```python
from build123d import *
from build123d.topology import SkipClean

# Parameters (mm, degrees)
SKETCH1_W           = 152
SKETCH1_H           = 65.5
BOSS_EXTRUDE1_DEPTH = 44
SKETCH2_W           = 142
SKETCH2_H           = 25.5
CUT_EXTRUDE1_DEPTH  = 39
SKETCH4_W           = 60
SKETCH4_H           = 30
CUT_EXTRUDE2_DEPTH  = 30
BOSS_EXTRUDE3_REACH = 158.9
SKETCH5_W           = 10
SKETCH5_H           = 15
SKETCH9_W           = 152
SKETCH9_H           = 44
BOSS_EXTRUDE4_DEPTH = 10
CUT_EXTRUDE5_DEPTH  = 41.5
SKETCH11_W          = 142
SKETCH11_H          = 39
CUT_EXTRUDE6_DEPTH  = 5
SKETCH16_W          = 77
SKETCH16_H          = 25
CUT_EXTRUDE8_DEPTH  = 39
SKETCH17_R          = 10.5
CUT_EXTRUDE9_DEPTH  = 5
SKETCH18_R          = 7.5
CUT_EXTRUDE10_DEPTH = 5
SKETCH20_W          = 75.5
SKETCH20_H          = 44
BOSS_EXTRUDE6_DEPTH = 15
SKETCH21_W          = 10
SKETCH21_H          = 55.5
CUT_EXTRUDE12_DEPTH = 39
SKETCH22_W          = 20
SKETCH22_H          = 20
SKETCH22_W_2        = 7.5
SKETCH22_H_2        = 25
CUT_EXTRUDE13_DEPTH = 5
CUT_EXTRUDE14_DEPTH = 3.5
SKETCH24_W          = 5
SKETCH24_H          = 6.5
BOSS_EXTRUDE7_DEPTH = 5
SKETCH24_3_W        = 3
SKETCH24_3_H        = 12
BOSS_EXTRUDE8_DEPTH = 2.5
CUT_EXTRUDE7_DEPTH  = 6
BOSS_EXTRUDE5_DEPTH = 3
SKETCH19_R          = 2.35
SKETCH19_R_2        = 2.5
CUT_EXTRUDE11_DEPTH = 6
BOSS_EXTRUDE9_DEPTH = 40
CHAMFER1_SIZE       = 0.3


with BuildPart() as part:
    # Sketch1 → Boss-Extrude1 (new body)
    with BuildSketch(Plane(origin=(0, 0, 0), x_dir=(1, 0, 0), z_dir=(0, 1, 0))):
        Rectangle(SKETCH1_W, SKETCH1_H)
    extrude(amount=BOSS_EXTRUDE1_DEPTH)

    # Sketch2 → Cut-Extrude1 (cut)
    with BuildSketch(Plane(origin=(0, 44, 0), x_dir=(1, 0, 0), z_dir=(0, 1, 0))):
        with Locations((0, -20)):
            Rectangle(SKETCH2_W, SKETCH2_H)
    extrude(amount=-CUT_EXTRUDE1_DEPTH, mode=Mode.SUBTRACT)

    # Sketch4 → Cut-Extrude2 (cut)
    with BuildSketch(Plane(origin=(0, 44, 0), x_dir=(1, 0, 0), z_dir=(0, 1, 0))):
        with Locations((41, 7.75)):
            Rectangle(SKETCH4_W, SKETCH4_H)
    extrude(amount=-CUT_EXTRUDE2_DEPTH, mode=Mode.SUBTRACT)

    # Boss-Extrude3: up to this face of the body (flat: up to its plane)
    boss_extrude3_end = Plane(part.part.faces().sort_by_distance((71, 26.637767221, 6.817102138))[0])
    # Sketch5 → Boss-Extrude3 (add, up to the picked face)
    with BuildSketch(Plane(origin=(-71, 0, 0), x_dir=(0, 0, -1), z_dir=(1, 0, 0)), mode=Mode.PRIVATE) as boss_extrude3_sk1:
        with Locations((-12.25, 36.5)):
            Rectangle(SKETCH5_W, SKETCH5_H)
    boss_extrude3_tool1 = split(extrude(boss_extrude3_sk1.sketch, amount=BOSS_EXTRUDE3_REACH, mode=Mode.PRIVATE), bisect_by=boss_extrude3_end, keep=Keep.BOTH, mode=Mode.PRIVATE)
    add(boss_extrude3_tool1.solids().sort_by(Axis((-71, 36.5, 12.25), (1, 0, 0)))[0])

    # Sketch9 → Boss-Extrude4 (add)
    with BuildSketch(Plane.XY.offset(32.75)):
        with Locations((0, 22)):
            Rectangle(SKETCH9_W, SKETCH9_H)
    extrude(amount=BOSS_EXTRUDE4_DEPTH)

    # Sketch10 → Cut-Extrude5 (cut)
    with BuildSketch(Plane(origin=(0, 44, 0), x_dir=(1, 0, 0), z_dir=(0, 1, 0))):
        Polygon((-73.5, -32.75), (-73.5, -37.75), (73.5, -37.75), (73.5, -32.75), (71, -32.75), (-71, -32.75), align=None)
    extrude(amount=-CUT_EXTRUDE5_DEPTH, mode=Mode.SUBTRACT)

    # Sketch11 → Cut-Extrude6 (cut)
    with BuildSketch(Plane.XY.offset(42.75)):
        with Locations((0, 24.5)):
            Rectangle(SKETCH11_W, SKETCH11_H)
    extrude(amount=-CUT_EXTRUDE6_DEPTH, mode=Mode.SUBTRACT)

    # Sketch16 → Cut-Extrude8 (cut)
    with BuildSketch(Plane(origin=(0, 44, 0), x_dir=(1, 0, 0), z_dir=(0, 1, 0))):
        with Locations((-32.5, 10.25)):
            Rectangle(SKETCH16_W, SKETCH16_H)
    extrude(amount=-CUT_EXTRUDE8_DEPTH, mode=Mode.SUBTRACT)

    # Sketch17 → Cut-Extrude9 (cut)
    with BuildSketch(Plane(origin=(-71, 0, 0), x_dir=(0, 0, -1), z_dir=(1, 0, 0))):
        with Locations((10.25, 29)):
            Circle(SKETCH17_R)
        with BuildLine():
            Line((7.5, 12), (13, 12))
            ThreePointArc((13, 12), (15, 10), (13, 8))
            Line((13, 8), (7.5, 8))
            ThreePointArc((7.5, 8), (5.5, 10), (7.5, 12))
        make_face()
    extrude(amount=-CUT_EXTRUDE9_DEPTH, mode=Mode.SUBTRACT)

    # Sketch18 → Cut-Extrude10 (cut)
    with BuildSketch(Plane(origin=(11, 0, 0), x_dir=(0, 0, -1), z_dir=(1, 0, 0))):
        with Locations((10.25, 24)):
            Circle(SKETCH18_R)
    extrude(amount=-CUT_EXTRUDE10_DEPTH, mode=Mode.SUBTRACT)

    # Sketch20 → Boss-Extrude6 (add)
    with BuildSketch(Plane(origin=(76, 0, 0), x_dir=(0, 0, -1), z_dir=(1, 0, 0))):
        with Locations((-5, 22)):
            Rectangle(SKETCH20_W, SKETCH20_H)
    extrude(amount=BOSS_EXTRUDE6_DEPTH)

    # Sketch21 → Cut-Extrude12 (cut)
    with BuildSketch(Plane(origin=(0, 44, 0), x_dir=(1, 0, 0), z_dir=(0, 1, 0))):
        with Locations((81, -5)):
            Rectangle(SKETCH21_W, SKETCH21_H)
    extrude(amount=-CUT_EXTRUDE12_DEPTH, mode=Mode.SUBTRACT)

    # Sketch22 → Cut-Extrude13 (cut)
    with BuildSketch(Plane(origin=(76, 0, 0), x_dir=(0, 0, -1), z_dir=(1, 0, 0))):
        with Locations((7.75, 29)):
            Rectangle(SKETCH22_W, SKETCH22_H)
        with Locations((-23.5, 22.5)):
            Rectangle(SKETCH22_W_2, SKETCH22_H_2)
    extrude(amount=-CUT_EXTRUDE13_DEPTH, mode=Mode.SUBTRACT)

    # Sketch23 → Cut-Extrude14 (cut)
    with BuildSketch(Plane(origin=(-71, 0, 0), x_dir=(0, 0, -1), z_dir=(1, 0, 0))):
        with BuildLine():
            ThreePointArc((7.5, 8), (5.5, 10), (7.5, 12))
            Line((7.5, 12), (4.25, 12))
            Line((4.25, 12), (4.25, 5))
            Line((4.25, 5), (16.25, 5))
            Line((16.25, 5), (16.25, 12))
            Line((16.25, 12), (13, 12))
            ThreePointArc((13, 12), (15, 10), (13, 8))
            Line((13, 8), (7.5, 8))
        make_face()
    extrude(amount=-CUT_EXTRUDE14_DEPTH, mode=Mode.SUBTRACT)

    # Sketch24 → Boss-Extrude7 (add)
    with BuildSketch(Plane(origin=(0, 5, 0), x_dir=(1, 0, 0), z_dir=(0, 1, 0))):
        with Locations((-68.5, 1)):
            Rectangle(SKETCH24_W, SKETCH24_H)
        with Locations((-68.5, 19.5)):
            Rectangle(SKETCH24_W, SKETCH24_H)
        Polygon((-45, -2.25), (-45, 4.25), (-48, 4.25), (-50, 4.25), (-50, -2.25), align=None)
        Polygon((-45, 22.75), (-50, 22.75), (-50, 16.25), (-48, 16.25), (-45, 16.25), align=None)
    extrude(amount=BOSS_EXTRUDE7_DEPTH)

    # Sketch24<3> → Boss-Extrude8 (add)
    with BuildSketch(Plane(origin=(0, 5, 0), x_dir=(1, 0, 0), z_dir=(0, 1, 0))):
        with Locations((-46.5, 10.25)):
            Rectangle(SKETCH24_3_W, SKETCH24_3_H)
    extrude(amount=BOSS_EXTRUDE8_DEPTH)

    # Sketch13 → Cut-Extrude7 (cut)
    with BuildSketch(Plane(origin=(0, 0, -32.75), x_dir=(-1, 0, 0), z_dir=(0, 0, -1))):
        with BuildLine():
            Line((-86, 34), (-86, 24))
            ThreePointArc((-86, 24), (-81, 19), (-76, 24))
            Line((-76, 24), (-76, 34))
            ThreePointArc((-76, 34), (-81, 39), (-86, 34))
        make_face()
        with BuildLine():
            Line((61, 34), (61, 24))
            ThreePointArc((61, 24), (66, 19), (71, 24))
            Line((71, 24), (71, 34))
            ThreePointArc((71, 34), (66, 39), (61, 34))
        make_face()
    extrude(amount=-CUT_EXTRUDE7_DEPTH, mode=Mode.SUBTRACT)

    # Sketch15 → Boss-Extrude5 (add)
    with SkipClean():  # the faces are left unmerged after this step: merging them gives an invalid solid
        with BuildSketch(Plane(origin=(0, 0, -32.75), x_dir=(-1, 0, 0), z_dir=(0, 0, -1))):
            with BuildLine():
                ThreePointArc((-76, 34), (-81, 39), (-86, 34))
                Line((-86, 34), (-86, 24))
                ThreePointArc((-86, 24), (-85.183300133, 26.738612788), (-83, 28.582575695))
                Line((-83, 28.582575695), (-83, 34))
                Line((-83, 34), (-79, 34))
                Line((-79, 34), (-79, 28.582575695))
                ThreePointArc((-79, 28.582575695), (-76.816699867, 26.738612788), (-76, 24))
                Line((-76, 24), (-76, 34))
            make_face()
            with BuildLine():
                ThreePointArc((71, 34), (66, 39), (61, 34))
                Line((61, 34), (61, 24))
                ThreePointArc((61, 24), (61.816699867, 26.738612788), (64, 28.582575695))
                Line((64, 28.582575695), (64, 34))
                Line((64, 34), (68, 34))
                Line((68, 34), (68, 28.582575695))
                ThreePointArc((68, 28.582575695), (70.183300133, 26.738612788), (71, 24))
                Line((71, 24), (71, 34))
            make_face()
        extrude(amount=-BOSS_EXTRUDE5_DEPTH)

    # Sketch19 → Cut-Extrude11 (cut)
    with SkipClean():  # the faces are left unmerged after this step: merging them gives an invalid solid
        with BuildSketch(Plane(origin=(0, 44, 0), x_dir=(1, 0, 0), z_dir=(0, 1, 0))):
            with Locations(Location((-66, -9.75, 0), (0, 0, 270))):
                Circle(SKETCH19_R)
            with Locations(Location((-51, 27.75, 0), (0, 0, 270))):
                Circle(SKETCH19_R)
            with Locations(Location((66, 27.75, 0), (0, 0, 270))):
                Circle(SKETCH19_R)
            with Locations(Location((81, -38.05, 0), (0, 0, 270))):
                Circle(SKETCH19_R_2)
        extrude(amount=-CUT_EXTRUDE11_DEPTH, mode=Mode.SUBTRACT)

    # Sketch25 → Boss-Extrude9 (add)
    with SkipClean():  # the faces are left unmerged after this step: merging them gives an invalid solid
        with BuildSketch(Plane.ZY.offset(-6)):
            with BuildLine():
                Line((-22.75, 21), (-22.75, 18.5))
                Line((-22.75, 18.5), (-16.25, 18.5))
                Line((-16.25, 18.5), (-16.25, 19.5))
                ThreePointArc((-16.25, 19.5), (-16.730477654, 20.224631227), (-17.123863542, 21))
                Line((-17.123863542, 21), (-22.75, 21))
            make_face()
            with BuildLine():
                Line((-4.25, 18.5), (2.25, 18.5))
                Line((2.25, 18.5), (2.25, 21))
                Line((2.25, 21), (-3.376136458, 21))
                ThreePointArc((-3.376136458, 21), (-3.769522346, 20.224631227), (-4.25, 19.5))
                Line((-4.25, 19.5), (-4.25, 18.5))
            make_face()
        extrude(amount=BOSS_EXTRUDE9_DEPTH)

    # Chamfer1
    chamfer1_edges = [part.edges().sort_by_distance(p)[0] for p in [
        (-66, 44, 7.4),
        (-51, 44, -30.1),
        (66, 44, -30.1),
        (81, 44, 35.55),
    ]]
    chamfer(chamfer1_edges, length=CHAMFER1_SIZE)


solid = part.part
```
Work out the finished part from the listing and answer in its coordinate system (mm). A direction names the side the tool comes from. Round coordinates to 2 decimals unless told otherwise and drop trailing zeros. Loops run counter-clockwise (first coordinate to the right, second up) from the corner with the lowest first, then second, coordinate; pieces in that order, holes last. Notation, with made-up numbers: M -13,-28.5 L -3,-28.5 A20 cw -3,-22.5 Z; hole C -38,75.25 d1. An arc over 180 degrees is marked long. One line per question, with ' | ' between items.
Q1. Find section C-C, the plane x = -58. Give the vertices of the cut face in (y, z).
Conclusion:
outline: M 0,-32.75 L 44,-32.75 L 44,-22.75 L 5,-22.75 L 5,2.25 L 44,2.25 L 44,17.25 L 29,17.25 L 29,7.25 L 5,7.25 L 5,32.75 L 2.5,32.75 L 2.5,37.75 L 5,37.75 L 5,42.75 L 0,42.75 Z
Q2. Find section B-B, the plane z = 30.5. Give the vertices of the cut face in (x, y).
Conclusion:
outline: M -76,0 L 91,0 L 91,44 L 86,44 L 86,5 L 76,5 L 76,44 L 71,44 L 71,5 L -71,5 L -71,44 L -76,44 Z
Q3. Find section D-D, the plane z = -10.25. State how many separate pieces and enclosed holes the cut face has, then the cut area to 3 significant figures.
Conclusion:
separate pieces: 5 | enclosed holes: 0 | area: 1,850 mm2
Q4. Consider line 1 along X through (y, z) = (9.5, 20.5); line 2 along X through (y, z) = (30, 3); line 3 along Y through (x, z) = (9.5, -10.25). Determine where each line is inside the solid, lowest interval first. Write a range as from..to.
Conclusion:
line 1: x = -76..-71, 71..76, 86..91 | line 2: x = -76..11, 71..76, 86..91 | line 3: y = 0..16.5, 31.5..44
Q5. Each of these flat-tipped pins is pushed along its axis until it touches: pin 1 Ø3 at (x, z) = (-35, -21.5) entering from +Y; pin 2 Ø1 at (y, z) = (28.5, -4.5) entering from -X; pin 3 Ø4.5 at (x, z) = (-11, -19) entering from +Y; pin 4 Ø12 at (x, y) = (-21, 28) entering from +Z. Where does it stop, or does it pass through?
Conclusion:
pin 1: stops at y = 44 | pin 2: stops at x = 6 | pin 3: stops at y = 21 | pin 4: stops at z = 17.25
Q6. A tool of negligible diameter and unlimited length cuts with its end or side. For faces 3 (the flat face through (-1, 5, 20)), 4 (the flat face through (74, 29, 2.25)), 5 (the flat face through (-1, 2.5, 35)), 6 (the flat face through (-66, 34, -31)), 7 (the flat face through (-71, 24, 40)), from which of +Z, -Z, +X, -X, +Y, -Y can it reach the whole face along a straight path? Write none if from no direction.
Conclusion:
face 3: +Z | face 4: none | face 5: +Y | face 6: -Z | face 7: +Z, +Y
Q7. The mould has two halves that part along X. Classify faces 1 (the flat face through (-66, 29, -26.75)), 2 (the cylindrical face through (-73.46, 39.41, -8.88)): +X half, -X half, draft (parallel to the pull), parting line (faces both ways), or undercut.
Conclusion:
face 1: undercut | face 2: draft
Q8. Find section A-A, the plane x = 66. Give the vertices of the cut face in (y, z), then the cut area to 3 significant figures.
Conclusion:
outline: M 0,-32.75 L 44,-32.75 L 44,-30.4 L 43.7,-30.1 L 38,-30.1 L 38,-25.4 L 43.7,-25.4 L 44,-25.1 L 44,-22.75 L 14,-22.75 L 14,7.25 L 5,7.25 L 5,32.75 L 2.5,32.75 L 2.5,37.75 L 5,37.75 L 5,42.75 L 0,42.75 Z; M 29,7.25 L 44,7.25 L 44,17.25 L 29,17.25 Z | area: 1,150 mm2
